```python
from build123d import *
from OCP.BRepFilletAPI import BRepFilletAPI_MakeChamfer

# Parameters (mm, degrees)
SZKIC1_R                    = 38.1
DODANIE_WYCI_GNI_CIE1_DEPTH = 30
SFAZOWANIE1_SIZE            = 15
SFAZOWANIE1_SIZE2           = 12.374392919
SFAZOWANIE2_SIZE            = 5


with BuildPart() as part:
    # Szkic1 → Dodanie-wyciągnięcie1 (new, symmetric)
    with BuildSketch(Plane(origin=(0, 0, 0), x_dir=(0, 0, -1), z_dir=(1, 0, 0))):
        with BuildLine():
            Line((0, -175), (-90, -175))
            Line((-90, -175), (-43.663859775, 10.884270741))
            ThreePointArc((-43.663859775, 10.884270741), (0, 45), (43.663859775, 10.884270741))
            Line((43.663859775, 10.884270741), (90, -175))
            Line((90, -175), (0, -175))
        make_face()
        Circle(SZKIC1_R, mode=Mode.SUBTRACT)
        with BuildLine():
            Line((0, -160), (70, -160))
            Line((70, -160), (36.631404611, -26.136950783))
            ThreePointArc((36.631404611, -26.136950783), (0, -45), (-36.631404611, -26.136950783))
            Line((-36.631404611, -26.136950783), (-70, -160))
            Line((-70, -160), (0, -160))
        make_face(mode=Mode.SUBTRACT)
    extrude(amount=DODANIE_WYCI_GNI_CIE1_DEPTH, both=True)

    # Sfazowanie1: one chamfer whose edges measure the first distance from different faces: ONE call of the kernel's chamfer builder (chamfer() names one face for all edges)
    sfazowanie1_edges_1 = [part.edges().sort_by_distance(p)[0] for p in [
        (0, -160, 70),
    ]]
    sfazowanie1_side_1 = [part.faces().sort_by_distance(p)[0] for p in [
        (0, -160, 0),
    ]]
    sfazowanie1_edges_2 = [part.edges().sort_by_distance(p)[0] for p in [
        (0, -160, -70),
    ]]
    sfazowanie1_side_2 = [part.faces().sort_by_distance(p)[0] for p in [
        (0, -93.068475391, -53.315702306),
    ]]
    sfazowanie1 = BRepFilletAPI_MakeChamfer(part.part.solid().wrapped)
    for e in sfazowanie1_edges_1:
        sfazowanie1.Add(SFAZOWANIE1_SIZE, SFAZOWANIE1_SIZE2, e.wrapped, sfazowanie1_side_1[0].wrapped)  # the first distance lies on this face
    for e in sfazowanie1_edges_2:
        sfazowanie1.Add(SFAZOWANIE1_SIZE, SFAZOWANIE1_SIZE2, e.wrapped, sfazowanie1_side_2[0].wrapped)  # the first distance lies on this face
    add(Compound.cast(sfazowanie1.Shape()), mode=Mode.REPLACE)

    # Sfazowanie2
    sfazowanie2_edges = [part.edges().sort_by_distance(p)[0] for p in [
        (30, -82.057864629, -66.831929887),
        (30, 45, 0),
        (30, -82.057864629, 66.831929887),
        (-30, -82.057864629, -66.831929887),
        (-30, 45, 0),
        (-30, -82.057864629, 66.831929887),
        (-30, -87.0649892, 51.819188497),
        (-30, -85.791165429, -51.501657182),
        (30, -85.791165429, -51.501657182),
        (30, -87.0649892, 51.819188497),
    ]]
    chamfer(sfazowanie2_edges, length=SFAZOWANIE2_SIZE)


solid = part.part
```
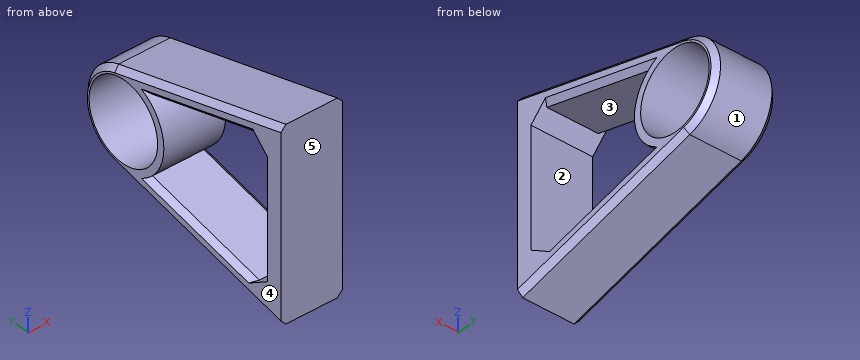
Source: CAD feature listing. Evaluate the final solid. Frame: model axes, mm. Face numbers are marked on the shaded views. A direction names the side the tool comes from. Coordinates: 2 decimals unless noted, no trailing zeros. Loops run counter-clockwise (first coordinate to the right, second up) from the corner with the lowest first, then second, coordinate; pieces in that order, holes last. Notation, with made-up numbers: (47, -27.75) -> (97, -27.75) arc R10 ccw to (97, -16.75) -> close; hole circle Ø1 at (46, 77). An arc over 180 degrees is marked (long way). One line per item, written item: value. Start each with the question number.
Q1. Section query D-D, the plane y = -87.5. Return the cut outline in (x, z).
Q2. Mould query, pull axis Y, two halves, no side actions, for the marked faces 3, 4 and 5. Classes: pulls with the +Y half, pulls with the -Y half, needs draft (parallel to the pull), parting line crosses it, or undercut.
Q3. Section query B-B, the plane x = -12.5. Return the cut outline in (y, z), and give its area (3 significant figures).
Q4. Contact query for flat-ended pins moving along their axis: P1, Ø1.5, axis at y = -108.5, z = -69.5, coming from the +X side; P2, Ø12, axis at x = -17, y = 22, coming from the -Z side; P3, Ø12, axis at x = -9.5, y = -72, coming from the +Z side. Output: stop coordinate, or through.
Q5. Line query: line 1 along Y through (x, z) = (8.5, 0); line 2 along Y through (x, z) = (-12, 34); line 3 along Z through (x, y) = (-12.5, -20.5). Output: solid intervals per line, ascending.
Q6. Set-up query: the marked faces 1 and 2. Return all of +Z, -Z, +X, -X, +Y, -Y with unobstructed straight access to the full face (end or side cutting, diameter ignored); none if empty.
Q7. Section query C-C, the plane y = -4. Return the cut outline in (x, z), and give its area (3 significant figures).
Q8. Section query A-A, the plane z = 0. Return the cut outline in (x, y), and give its area (3 significant figures).
Results:
1. outline: (-30, -63.04) -> (-25, -68.19) -> (25, -68.19) -> (30, -63.04) -> (30, -57.08) -> (25, -51.93) -> (-25, -51.93) -> (-30, -57.08) -> close; (-30, 57.08) -> (-25, 51.93) -> (25, 51.93) -> (30, 57.08) -> (30, 63.04) -> (25, 68.19) -> (-25, 68.19) -> (-30, 63.04) -> close
2. face 3: undercut
2. face 4: needs draft
2. face 5: pulls with the -Y half
3. outline: (-175, -90) -> (10.88, -43.66) arc R45 ccw to (10.88, 43.66) -> (-175, 90) -> close; hole (-160, -57.63) -> (-145.45, -66.37) -> (-26.14, -36.63) arc R45 cw to (-26.14, 36.63) -> (-147.99, 67.01) -> (-160, 55) -> close; hole circle Ø76.2 at (0, 0)
3. area: 9,370 mm^2
4. P1: x = 29.56
4. P2: z = -42.06
4. P3: z = 65.82
5. line 1: -175 to -160, -45 to -38.1, 38.1 to 45
5. line 2: -175 to -160, -29.48 to -17.19, 17.19 to 29.48
5. line 3: -51.49 to -32.11, 32.11 to 51.49
6. face 1: +X, -X, +Y
6. face 2: +X, -X
7. outline: (-30, -42.22) -> (-25, -47.37) -> (25, -47.37) -> (30, -42.22) -> (30, -37.89) -> (-30, -37.89) -> close; (-30, 37.89) -> (30, 37.89) -> (30, 42.22) -> (25, 47.37) -> (-25, 47.37) -> (-30, 42.22) -> close
7. area: 1,090 mm^2
8. outline: (-30, -175) -> (30, -175) -> (30, -160) -> (-30, -160) -> close; (-30, -45) -> (30, -45) -> (30, -38.1) -> (-30, -38.1) -> close; (-30, 38.1) -> (30, 38.1) -> (30, 40) -> (25, 45) -> (-25, 45) -> (-30, 40) -> close
8. area: 1,700 mm^2
